Part model, mm, in its own coordinate system. A direction names the side the tool comes from. Round coordinates to 2 decimals unless told otherwise and drop trailing zeros. Loops run counter-clockwise (first coordinate to the right, second up) from the corner with the lowest first, then second, coordinate; pieces in that order, holes last. Notation, with made-up numbers: (-4.75, 48.25) -> (48.25, 48.25) arc R25 cw to (48.25, 79.25) -> close; hole circle Ø11 at (88.5, 46.25). An arc over 180 degrees is marked (long way). Use a Markdown table: item, result. Add a question column.
Item 1: Cut at B-B, the plane y = -4. List the corners of the cut face in (x, z), plus the area to 3 significant figures.
Item 2: Flat gauge pin, fed straight in: pin 1 (4.5 mm diameter, centred on x = -19, z = 6.5, fed in from +Y). Where does the tip first touch, or does it go through?
Item 3: Two-plate mould, pull along X, no slides. Class faces 1 (the face through (0, 15, 0)), 2 (the face through (-13.298, -13.87, 15.566)): pulls with the +X half, pulls with the -X half, needs draft (parallel to the pull), parting line crosses it, or undercut.
Item 4: Cut at C-C, the plane x = 0. List the corners of the cut face in (y, z), plus the area to 3 significant figures.
Item 5: Which spindle directions (+Z, -Z, +X, -X, +Y, -Y) get a long thin tool onto all of the face, cutting with end or side? Do faces 3 (the face through (-20.385, 12.303, 30.73)), 4 (the face through (-11.11, -14.65, 26.73)), 5 (the face through (8.5, -16, 18)), 6 (the face through (-0.49, 14.04, 18.18)), 7 (the face through (-16, -20, 18)). Say none if no direction does.
Item 6: Probe line 1 (X direction, y = 16.25, z = 6.5) (3 decimals); line 2 (Z direction, x = -19, y = 16) (1 decimal); line 3 (Y direction, x = 15, z = 29). List the from-to ranges inside material, lowest first. Write a range as [from, to].
Item 7: Cut at A-A, the plane y = 18.5. State how many separate pieces and enclosed holes the cut face has, plus the area to 3 significant figures.
Autodesk Inventor part; units mm, degrees
ref_plane "YZ Plane" through (0, 0, 0) normal (1, 0, 0) x (0, 1, 0)
ref_plane "XZ Plane" through (0, 0, 0) normal (0, 1, 0) x (-1, 0, 0)
ref_plane "XY Plane" through (0, 0, 0) normal (0, 0, 1) x (1, 0, 0)
sketch "Sketch1" plane through (0, 0, 0) normal (0, 0, 1) x (1, 0, 0)
  line L0 (-24, 20) -> (24, 20)
  line L1 (-24, 20) -> (-24, -20)
  line L2 (-24, -20) -> (-8.5, -20)
  line L3 (24, 20) -> (24, -20)
  line L4 (24, -20) -> (8.5, -20)
  arc A0 (8.5, -11.1872) -> (-8.5, -11.1872) centre (0, 0) ccw
  line L5 (-8.5, -20) -> (-8.5, -11.1872)
  line L6 (8.5, -20) -> (8.5, -11.1872)
  point P0 (0, 20)
  point P1 (-24, 0)
  dimension "d0" = 48
  dimension "d1" = 40
  dimension "d2" = 17
  dimension "d3" = 15.5
  dimension "d4" = 40
  dimension "d6" = 14.05
  dimension "d70" = 8.8128
extrude "Extrusion1" add sketch "Sketch1" along normal blind 36.8695
sketch "Sketch2" plane through (0, 0, 36.8695) normal (0, 0, 1) x (1, 0, 0)
  line L0 (-24, 20) -> (-24, -20)
  arc A0 (8.5, -11.1872) -> (-8.5, -11.1872) centre (0, 0) ccw
  circle A1 centre (0, 0) radius 19 construction
  point P0 (-19, 0)
  point P1 (-24, 0)
  point P2 (-13.435, -13.435)
  point P3 (-13.435, 13.435)
  point P4 (13.435, 13.435)
  point P5 (19, 0)
  point P6 (13.435, -13.435)
  dimension "d9" = 38
  dimension "d12" = 45
  dimension "d16" = 45
  dimension "d18" = 45
  dimension "d19" = 45
hole "Hole1" at (-19, 0, 36.8695) at (-13.435, -13.435, 36.8695) at (-13.435, 13.435, 36.8695) at (13.435, 13.435, 36.8695) at (19, 0, 36.8695) at (13.435, -13.435, 36.8695) direction (0, 0, -1) diameter 5.25 depth 20 tip angle 118
thread "Thread1"
thread "Thread2"
thread "Thread3"
thread "Thread4"
thread "Thread5"
thread "Thread6"
sketch "Sketch3" plane through (-24, 20, 0) normal (0, 1, 0) x (1, 0, 0)
  line L0 (0, 0) -> (48, 0)
  line L1 (0, 0) -> (0, -36.8695)
  point P0 (24, 0)
  point P1 (5, -6.5)
  point P2 (43, -6.5)
  point P3 (5, -28.5)
  point P4 (43, -28.5)
  dimension "d41" = 38
  dimension "d44" = 22
  dimension "d47" = 6.5
  dimension "d48" = 5
hole "Hole2" at (-19, 20, 6.5) at (19, 20, 6.5) at (-19, 20, 28.5) at (19, 20, 28.5) direction (0, -1, 0) diameter 5.25 depth 17
thread "Thread7"
thread "Thread8"
thread "Thread9"
thread "Thread10"
sketch "Sketch4" plane through (-24, 20, 0) normal (0, 1, 0) x (1, 0, 0)
  circle A0 centre (5, -28.5) radius 2.625
  circle A1 centre (5, -6.5) radius 2.625
  circle A2 centre (43, -6.5) radius 2.625
  circle A3 centre (43, -28.5) radius 2.625
  line L0 (0, 0) -> (48, 0)
  line L1 (0, 0) -> (0, -36.8695)
  line L2 (48, -36.8695) -> (0, -36.8695)
  line L3 (48, 0) -> (48, -36.8695)
  point P0 (24, 0)
  dimension "d64" = 48
  dimension "d65" = 36.8695
  dimension "d66" = 38
  dimension "d67" = 22
  dimension "d68" = 5
  dimension "d69" = 6.5
sketch "Sketch5" plane through (-24, 20, 0) normal (0, 1, 0) x (1, 0, 0)
  circle A0 centre (5, -28.5) radius 2.625
  circle A1 centre (5, -6.5) radius 2.625
  circle A2 centre (43, -6.5) radius 2.625
  circle A3 centre (43, -28.5) radius 2.625
  line L0 (0, 0) -> (48, 0)
  line L1 (0, 0) -> (0, -36.8695)
  line L2 (48, -36.8695) -> (0, -36.8695)
  line L3 (48, 0) -> (48, -36.8695)
  point P0 (24, 0)
extrude "Extrusion2" add sketch "Sketch5" along normal blind 1.8695
equation "\"d3\" = -0.5 * d2 + 0.5 * d0"
equation "\"d4\" = d1"
properties part number "HD16"
A:
| question | item | result |
|---|---|---|
| 1 | outline | (-24, 0) -> (-13.47, 0) -> (-13.47, 36.87) -> (-24, 36.87) -> close; (13.47, 0) -> (24, 0) -> (24, 36.87) -> (13.47, 36.87) -> close |
| 1 | area | 777 mm^2 |
| 2 | pin 1 | stops at y = 3 |
| 3 | face 1 | needs draft |
| 3 | face 2 | undercut |
| 4 | outline | (14.05, 0) -> (21.87, 0) -> (21.87, 36.87) -> (14.05, 36.87) -> close |
| 4 | area | 288 mm^2 |
| 5 | face 3 | +Y |
| 5 | face 4 | +Z |
| 5 | face 5 | +Z, -Z, -Y |
| 5 | face 6 | +Z, -Z |
| 5 | face 7 | +Z, -Z, +X, -X, -Y |
| 6 | line 1 | x = [-24, -21.625], [-16.375, 16.375], [21.625, 24] |
| 6 | line 2 | z = [0, 3.9], [9.1, 25.9], [31.1, 36.9] |
| 6 | line 3 | y = [-20, -15.54], [-11.33, 11.33], [15.54, 21.87] |
| 7 | separate pieces | 1 |
| 7 | enclosed holes | 4 |
| 7 | area | 1,680 mm^2 |
